For this review, take the finished solid that the model builds, in its own axes (mm). A direction names the side the tool comes from. Round coordinates to 2 decimals unless told otherwise and drop trailing zeros. Order: outer loops, then holes, each group sorted by start corner. A loop starts at its lowest first (then second) coordinate and runs counter-clockwise, first axis right, second up. Notation, with made-up numbers: M 55,29 L 84,29 A30 cw 84,68 Z; hole C -19,-23.5 d2. An arc over 180 degrees is marked long. Write item = value, one per line. Start each with the question number.
from build123d import *

# Parameters (mm, degrees)
SKETCH1_R           = 22
SKETCH1_R_2         = 2.2
BOSS_EXTRUDE1_DEPTH = 1
SKETCH2_R           = 2
SKETCH2_R_2         = 2.2
BOSS_EXTRUDE2_DEPTH = 6
SKETCH3_W           = 25
SKETCH3_H           = 15
SKETCH3_R           = 2.2
BOSS_EXTRUDE3_DEPTH = 8
CUT_EXTRUDE1_DEPTH  = 16
SKETCH5_R           = 3.55
CUT_EXTRUDE2_DEPTH  = 4
FILLET1_R           = 3
SKETCH6_R           = 3.75
CUT_EXTRUDE3_DEPTH  = 4.5


with BuildPart() as part:
    # Sketch1 → Boss-Extrude1 (new body)
    with BuildSketch(Plane.XY):
        Circle(SKETCH1_R)
        with Locations((10.606601718, 10.606601718)):
            Circle(SKETCH1_R_2, mode=Mode.SUBTRACT)
        with Locations((10.606601718, -10.606601718)):
            Circle(SKETCH1_R_2, mode=Mode.SUBTRACT)
        with Locations((-10.606601718, -10.606601718)):
            Circle(SKETCH1_R_2, mode=Mode.SUBTRACT)
        with Locations((-10.606601718, 10.606601718)):
            Circle(SKETCH1_R_2, mode=Mode.SUBTRACT)
    extrude(amount=BOSS_EXTRUDE1_DEPTH)

    # Sketch2 → Boss-Extrude2 (add)
    with BuildSketch(Plane.XY.offset(1)):
        with BuildLine():
            Line((-48.055, -75), (-55, -95))
            Line((-55, -95), (-30, -95))
            Line((-30, -95), (-30, -65))
            Line((-30, -65), (30, -65))
            Line((30, -65), (30, -95))
            Line((30, -95), (55, -95))
            Line((55, -95), (48.055, -75))
            Line((48.055, -75), (20.881333045, 6.926032793))
            ThreePointArc((20.881333045, 6.926032793), (0, 22), (-20.881333045, 6.926032793))
            Line((-20.881333045, 6.926032793), (-48.055, -75))
        make_face()
        with Locations((-30, -55)):
            Circle(SKETCH2_R, mode=Mode.SUBTRACT)
        with Locations((30, -55)):
            Circle(SKETCH2_R, mode=Mode.SUBTRACT)
        with Locations((-10.606601718, -10.606601718)):
            Circle(SKETCH2_R_2, mode=Mode.SUBTRACT)
        with Locations((-10.606601718, 10.606601718)):
            Circle(SKETCH2_R_2, mode=Mode.SUBTRACT)
        with Locations((10.606601718, -10.606601718)):
            Circle(SKETCH2_R_2, mode=Mode.SUBTRACT)
        with Locations((10.606601718, 10.606601718)):
            Circle(SKETCH2_R_2, mode=Mode.SUBTRACT)
    extrude(amount=BOSS_EXTRUDE2_DEPTH)

    # Sketch3 → Boss-Extrude3 (add)
    with BuildSketch(Plane(origin=(0, -95, 0), x_dir=(-1, 0, 0), z_dir=(0, -1, 0))):
        with Locations((-42.5, 6.5)):
            Rectangle(SKETCH3_W, SKETCH3_H)
        with Locations((-35, 6.5)):
            Circle(SKETCH3_R, mode=Mode.SUBTRACT)
        with Locations((-50, 6.5)):
            Circle(SKETCH3_R, mode=Mode.SUBTRACT)
        with Locations((42.5, 6.5)):
            Rectangle(SKETCH3_W, SKETCH3_H)
        with Locations((50, 6.5)):
            Circle(SKETCH3_R, mode=Mode.SUBTRACT)
        with Locations((35, 6.5)):
            Circle(SKETCH3_R, mode=Mode.SUBTRACT)
    extrude(amount=-BOSS_EXTRUDE3_DEPTH)

    # Sketch4 → Cut-Extrude1 (cut, through all)
    with BuildSketch(Plane.XY.offset(1)):
        Polygon((-55, -95), (-52.222, -87), (-55, -87), align=None)
        Polygon((55, -95), (55, -87), (52.222, -87), align=None)
    extrude(amount=-CUT_EXTRUDE1_DEPTH, mode=Mode.SUBTRACT)

    # Sketch5 → Cut-Extrude2 (cut)
    with BuildSketch(Plane(origin=(0, -87, 0), x_dir=(1, 0, 0), z_dir=(0, 1, 0))):
        with Locations((-50, 6.5)):
            Circle(SKETCH5_R)
        with Locations((-35, 6.5)):
            Circle(SKETCH5_R)
        with Locations((35, 6.5)):
            Circle(SKETCH5_R)
        with Locations((50, 6.5)):
            Circle(SKETCH5_R)
    extrude(amount=-CUT_EXTRUDE2_DEPTH, mode=Mode.SUBTRACT)

    # Fillet1
    fillet1_edges = [part.edges().sort_by_distance(p)[0] for p in [
        (-53.611, -91, -14),
        (53.611, -91, -14),
        (30, -65, 4),
        (-30, -65, 4),
        (30, -91, -14),
        (-30, -91, -14),
    ]]
    fillet(fillet1_edges, radius=FILLET1_R)

    # Sketch6 → Cut-Extrude3 (cut)
    with BuildSketch(Plane.XY.offset(7)):
        with Locations((-10.606601718, 10.606601718)):
            Circle(SKETCH6_R)
        with Locations((10.606601718, 10.606601718)):
            Circle(SKETCH6_R)
        with Locations((10.606601718, -10.606601718)):
            Circle(SKETCH6_R)
        with Locations((-10.606601718, -10.606601718)):
            Circle(SKETCH6_R)
    extrude(amount=-CUT_EXTRUDE3_DEPTH, mode=Mode.SUBTRACT)


solid = part.part
(1) For line 1 along Z through (x, y) = (50, -93); line 2 along Z through (x, y) = (-50, -89.6); line 3 along X through (y, z) = (11, 4), list the stretches that pass through material, from the lowest coordinate up.
(2) Insertion check: pin 1 (2 mm diameter, centred on x = 36, y = -69, fed in from -Z); pin 2 (5.5 mm diameter, centred on x = -10.61, y = 10.61, fed in from +Z); pin 3 (2 mm diameter, centred on x = 49, z = -7.5, fed in from +Y); pin 4 (5.5 mm diameter, centred on x = 35, z = -6.5, fed in from -Y). Each pin has a flat end and moves straight along its axis. Give the tip position at first contact, or say it passes through.
(3) We need section D-D, the plane x = 35. Write out the cut boundary in (y, z).
(4) For faces 4 (the flat face through (30, -85, 2)), 5 (the cylindrical face through (31.453, -88.972, -6.656)), 6 (the cylindrical face through (-30.86, -90.94, -13.1)), 7 (the flat face through (34.66, -34.61, 3.96)), 8 (the cylindrical face through (14.07, 9.17, 4.78)), list the 3-axis set-ups (+Z, -Z, +X, -X, +Y, -Y) from which the entire face can be reached by the end or side of a thin tool; tool diameter is ignored.
(5) We need section A-A, the plane y = -55. Write out the cut boundary in (x, z).
(6) We need section C-C, the plane z = 4.5. Write out the cut boundary in (x, y) (3 decimals), then the cut area to 3 significant figures.
(7) We need section B-B, the plane x = -10. Write out the cut boundary in (y, z), then the cut area to 3 significant figures.
(8) Draft analysis for pull direction Y (two halves, no side actions). For faces 1 (the flat face through (-52.25, -87.08, 1.87)), 2 (the flat face through (-1, -50, 1)), 3 (the cylindrical face through (-28.092, -54.399, 3.958)), state which applies: released by +Y, released by -Y, zero draft, split by the parting line, or undercut.
Values:
q1.line_1 = -14 to -8.7, -4.3 to 7
q1.line_2 = -14 to -10.05, -2.95 to 7
q1.line_3 = -19.05 to -14.34, -6.88 to 6.88, 14.34 to 19.05
q2.pin_1 = 1
q2.pin_2 = 2.5
q2.pin_3 = -91
q2.pin_4 = -95
q3.outline = M -95,-14 L -87,-14 L -87,-10.05 L -91,-10.05 L -91,-8.7 L -95,-8.7 Z; M -95,-4.3 L -91,-4.3 L -91,-2.95 L -87,-2.95 L -87,1 L -35.64,1 L -35.64,7 L -95,7 Z
q4.face_4 = +Z, -Z, -Y
q4.face_5 = +Y
q4.face_6 = -Z, +Y, -Y
q4.face_7 = +Z, -Z, +X, +Y
q4.face_8 = +Z
q5.outline = M -41.42,1 L -32,1 L -32,7 L -41.42,7 Z; M -28,1 L 28,1 L 28,7 L -28,7 Z; M 32,1 L 41.42,1 L 41.42,7 L 32,7 Z
q6.outline = M -55,-95 L -30,-95 L -30,-68 A3 cw -27,-65 L 27,-65 A3 cw 30,-68 L 30,-95 L 55,-95 L 48.055,-75 L 20.881,6.926 A22 ccw -20.881,6.926 L -48.055,-75 Z; hole C -30,-55 d4; hole C -10.607,-10.607 d7.5; hole C -10.607,10.607 d7.5; hole C 10.607,-10.607 d7.5; hole C 10.607,10.607 d7.5; hole C 30,-55 d4
q6.area = 6,170 mm²
q7.outline = M -65,1 L -19.6,1 L -19.6,0 L -12.72,0 L -12.72,2.5 L -14.31,2.5 L -14.31,7 L -65,7 Z; M -8.49,0 L 8.49,0 L 8.49,2.5 L 6.91,2.5 L 6.91,7 L -6.91,7 L -6.91,2.5 L -8.49,2.5 Z; M 12.72,0 L 19.6,0 L 19.6,7 L 14.31,7 L 14.31,2.5 L 12.72,2.5 Z
q7.area = 459 mm²
q8.face_1 = released by +Y
q8.face_2 = zero draft
q8.face_3 = undercut
